from build123d import *

# Parameters (mm, degrees)
SKETCH1_W           = 128.3
SKETCH1_H           = 64.29
BOSS_EXTRUDE1_DEPTH = 5
SKETCH2_R           = 1.1
CUT_EXTRUDE1_DEPTH  = 6
SKETCH3_W           = 72
SKETCH3_H           = 25.13
CUT_EXTRUDE2_DEPTH  = 6


with BuildPart() as part:
    # Sketch1 → Boss-Extrude1 (new body)
    with BuildSketch(Plane(origin=(0, 0, 0), x_dir=(1, 0, 0), z_dir=(0, 1, 0))):
        with Locations((-64.15, 32.145)):
            Rectangle(SKETCH1_W, SKETCH1_H)
    extrude(amount=BOSS_EXTRUDE1_DEPTH)

    # Sketch2 → Cut-Extrude1 (cut, through all)
    with BuildSketch(Plane(origin=(0, 0, 0), x_dir=(-1, 0, 0), z_dir=(0, -1, 0))):
        with Locations((125.8, 2.5)):
            Circle(SKETCH2_R)
        with Locations((125.8, 61.79)):
            Circle(SKETCH2_R)
        with Locations((2.5, 2.5)):
            Circle(SKETCH2_R)
        with Locations((2.5, 61.79)):
            Circle(SKETCH2_R)
    extrude(amount=-CUT_EXTRUDE1_DEPTH, mode=Mode.SUBTRACT)

    # Sketch3 → Cut-Extrude2 (cut, through all)
    with BuildSketch(Plane.XZ):
        with Locations((-77.3, -27.565)):
            Rectangle(SKETCH3_W, SKETCH3_H)
    extrude(amount=-CUT_EXTRUDE2_DEPTH, mode=Mode.SUBTRACT)


solid = part.part
Input: part model. Units: mm. Frame: model coordinates. A direction names the side the tool comes from. Coordinates: 2 decimals unless noted, no trailing zeros. Loops run counter-clockwise (first coordinate to the right, second up) from the corner with the lowest first, then second, coordinate; pieces in that order, holes last. Notation, with made-up numbers: (-4, -39.75) - (16, -39.75) arc R24 ccw to (16, -29.75) - close; hole circle Ø11 at (69.5, -17). An arc over 180 degrees is marked (long way). Answer in a Markdown table with one row per item. Add a question column.
Item 1: Contact query for a flat-ended pin moving along its axis: P1, Ø1.8, axis at x = -125.8, z = -61.79, coming from the -Y side. Output: stop coordinate, or through.
Item 2: Access query for faces 1 (the flat face through (-65, 5, -47)), 2 (the flat face through (-78, 2, -40.13)). Directions: +Z, -Z, +X, -X, +Y, -Y. A direction counts if a zero-diameter tool reaches every point of the face in a straight line with its end or side. Return the directions, or none.
Item 3: Line query: line 1 along Z through (x, y) = (-2.5, 2.15); line 2 along X through (y, z) = (0.35, -27.5); line 3 along Z through (x, y) = (-96, 0.3). Output: solid intervals per line, ascending. Write a range as [from, to].
Item 4: Mould query, pull axis X, two halves, no side actions, for faces 3 (the flat face through (-128.3, 2, -32)), 4 (the flat face through (-65, 2, -64.29)), 5 (the flat face through (-78, 2, -15)). Classes: released by +X, released by -X, zero draft, split by the parting line, or undercut.
Item 5: Section query B-B on y = 1.8. Return the cut outline in (x, z), then the cut area to 3 significant figures.
Item 6: Section query C-C on z = -28. Return the cut outline in (x, y).
Item 7: Section query A-A on x = -70. Return the cut outline in (y, z).
Recorded:
| question | item | result |
|---|---|---|
| 1 | P1 | through |
| 2 | face 1 | +Z, -Z, +X, -X, +Y |
| 2 | face 2 | +Y, -Y |
| 3 | line 1 | [-64.29, -62.89], [-60.69, -3.6], [-1.4, 0] |
| 3 | line 2 | [-128.3, -113.3], [-41.3, 0] |
| 3 | line 3 | [-64.29, -40.13], [-15, 0] |
| 4 | face 3 | released by -X |
| 4 | face 4 | zero draft |
| 4 | face 5 | undercut |
| 5 | outline | (-128.3, -64.29) - (0, -64.29) - (0, 0) - (-128.3, 0) - close; hole circle Ø2.2 at (-125.8, -61.79); hole circle Ø2.2 at (-125.8, -2.5); hole (-113.3, -40.13) - (-41.3, -40.13) - (-41.3, -15) - (-113.3, -15) - close; hole circle Ø2.2 at (-2.5, -61.79); hole circle Ø2.2 at (-2.5, -2.5) |
| 5 | area | 6,420 mm^2 |
| 6 | outline | (-128.3, 0) - (-113.3, 0) - (-113.3, 5) - (-128.3, 5) - close; (-41.3, 0) - (0, 0) - (0, 5) - (-41.3, 5) - close |
| 7 | outline | (0, -64.29) - (5, -64.29) - (5, -40.13) - (0, -40.13) - close; (0, -15) - (5, -15) - (5, 0) - (0, 0) - close |
